```python
from build123d import *

# Parameters (mm, degrees)
SKETCH1_W               = 40
SKETCH1_H               = 20
BOSS_EXTRUDE1_DEPTH     = 36.6
SKETCH2_W               = 18
SKETCH2_H               = 2.6
BOSS_EXTRUDE2_DEPTH     = 7.25
SKETCH3_R               = 2.25
CUT_EXTRUDE1_DEPTH      = 42.17283692
MIRROR3_COPY_1_SKETCH_R = 2.25
MIRROR3_COPY_1_DEPTH    = 42.17283692
FILLET1_R               = 1
CHAMFER1_SIZE           = 1


with BuildPart() as part:
    # Sketch1 → Boss-Extrude1 (new body)
    with BuildSketch(Plane(origin=(0, 0, 0), x_dir=(1, 0, 0), z_dir=(0, 1, 0))):
        Rectangle(SKETCH1_W, SKETCH1_H)
    extrude(amount=BOSS_EXTRUDE1_DEPTH)

    # Sketch2 → Boss-Extrude2 (add)
    with BuildSketch(Plane(origin=(20, 0, 0), x_dir=(0, 0, -1), z_dir=(1, 0, 0))):
        with Locations((0, 27.9)):
            Rectangle(SKETCH2_W, SKETCH2_H)
    boss_extrude2 = extrude(amount=BOSS_EXTRUDE2_DEPTH)

    # Sketch3 → Cut-Extrude1 (cut, through all)
    with BuildSketch(Plane(origin=(0, 29.2, 0), x_dir=(1, 0, 0), z_dir=(0, 1, 0))):
        with Locations(Location((24.75, 5, 0), (0, 0, 270))):
            Circle(SKETCH3_R)
    cut_extrude1 = extrude(amount=-CUT_EXTRUDE1_DEPTH, mode=Mode.SUBTRACT)

    # Mirror2: Cut-Extrude1 across plane
    add(cut_extrude1.mirror(Plane.XY), mode=Mode.SUBTRACT)

    # Mirror3: Boss-Extrude2, Cut-Extrude1 across plane
    add(boss_extrude2.mirror(Plane(origin=(0, 0, 0), x_dir=(0, 0, 1), z_dir=(1, 0, 0))))
    add(cut_extrude1.mirror(Plane(origin=(0, 0, 0), x_dir=(0, 0, 1), z_dir=(1, 0, 0))), mode=Mode.SUBTRACT)

    # Mirror3 copy 1 sketch → Mirror3 copy 1 (cut, through all)
    with BuildSketch(Plane(origin=(0, 29.2, 0), x_dir=(-1, 0, 0), z_dir=(0, 1, 0))):
        with Locations(Location((24.75, 5, 0), (0, 0, 270))):
            Circle(MIRROR3_COPY_1_SKETCH_R)
    extrude(amount=-MIRROR3_COPY_1_DEPTH, mode=Mode.SUBTRACT)

    # Fillet1
    fillet1_edges = [part.edges().sort_by_distance(p)[0] for p in [
        (20, 18.3, 10),
        (-20, 18.3, 10),
        (-20, 18.3, -10),
        (20, 18.3, -10),
    ]]
    fillet(fillet1_edges, radius=FILLET1_R - 0.0001)  # a hair under: the kernel refuses the full size

    # Chamfer1
    chamfer1_edges = [part.edges().sort_by_distance(p)[0] for p in [
        (20, 0, 0),
        (0, 0, 10),
        (-20, 0, 0),
        (0, 0, -10),
        (-19.707136071, 0, 9.707136071),
        (-19.707136071, 0, -9.707136071),
        (19.707136071, 0, -9.707136071),
        (19.707136071, 0, 9.707136071),
    ]]
    chamfer(chamfer1_edges, length=CHAMFER1_SIZE - 0.0001)  # a hair under: the kernel refuses the full size


solid = part.part
```
Can you work these out from the model? Positions are in its coordinate system, mm. A direction names the side the tool comes from. Coordinates: 2 decimals unless noted, no trailing zeros. Loops run counter-clockwise (first coordinate to the right, second up) from the corner with the lowest first, then second, coordinate; pieces in that order, holes last.
Item 1: Please list where these lines run through material, in increasing order: L1, parallel to X at y = 27.85, z = 5; L2, parallel to Z at x = -24.75, y = 27.8; L3, parallel to Z at x = -24, y = 27.
Answers below:
L1: x = -27.25 to -27, -22.5 to 22.5, 27 to 27.25
L2: z = -9 to -7.25, -2.75 to 2.75, 7.25 to 9
L3: z = -9 to -7.12, -2.88 to 2.88, 7.12 to 9
Item 2: Suppose I cut it at C-C (y = 33.5). Please give me the cut outline in (x, z), then the cut area to 3 significant figures.
Answers below:
outline: (-20, -9) arc R1 ccw to (-19, -10) - (19, -10) arc R1 ccw to (20, -9) - (20, 9) arc R1 ccw to (19, 10) - (-19, 10) arc R1 ccw to (-20, 9) - close
area: 799 mm2
Item 3: I'm going to push flat-ended pins straight in: pin 1 (12 mm diameter, centred on y = 10, z = 6, fed in from +X); pin 2 (1 mm diameter, centred on y = 7.5, z = 1, fed in from -X); pin 3 (3.5 mm diameter, centred on x = -23, z = 3.5, fed in from +Y). Where does each tip first touch, or does it pass through?
Answers below:
pin 1: stops at x = 20
pin 2: stops at x = -20
pin 3: stops at y = 29.2
Item 4: Suppose I cut it at D-D (z = 0). Please give me the cut outline in (x, y).
Answers below:
outline: (-27.25, 26.6) - (-20, 26.6) - (-20, 1) - (-19, 0) - (19, 0) - (20, 1) - (20, 26.6) - (27.25, 26.6) - (27.25, 29.2) - (20, 29.2) - (20, 36.6) - (-20, 36.6) - (-20, 29.2) - (-27.25, 29.2) - close
Item 5: Suppose I cut it at A-A (z = -5). Please give me the cut outline in (x, y).
Answers below:
outline: (-27.25, 26.6) - (-27, 26.6) - (-27, 29.2) - (-27.25, 29.2) - close; (-22.5, 26.6) - (-20, 26.6) - (-20, 1) - (-19, 0) - (19, 0) - (20, 1) - (20, 26.6) - (22.5, 26.6) - (22.5, 29.2) - (20, 29.2) - (20, 36.6) - (-20, 36.6) - (-20, 29.2) - (-22.5, 29.2) - close; (27, 26.6) - (27.25, 26.6) - (27.25, 29.2) - (27, 29.2) - close
Item 6: Which directions (+Z, -Z, +X, -X, +Y, -Y) give clear straight access to the entire face, cutting with the end or side of a thin tool? Please do faces 4 (the face through (24, 28, -9)), 5 (the face through (24, 28, 9)), 6 (the face through (-24, 28, 9)), 7 (the face through (24, 29.2, 0)), 8 (the face through (-24, 29.2, 0)).
Answers below:
face 4: -Z, +X, +Y, -Y
face 5: +Z, +X, +Y, -Y
face 6: +Z, -X, +Y, -Y
face 7: +Z, -Z, +X, +Y
face 8: +Z, -Z, -X, +Y
Item 7: Suppose I cut it at B-B (x = 24.75). Please give me the cut outline in (y, z), then the cut area to 3 significant figures.
Answers below:
outline: (26.6, -9) - (29.2, -9) - (29.2, -7.25) - (26.6, -7.25) - close; (26.6, -2.75) - (29.2, -2.75) - (29.2, 2.75) - (26.6, 2.75) - close; (26.6, 7.25) - (29.2, 7.25) - (29.2, 9) - (26.6, 9) - close
area: 23.4 mm2
Item 8: If we mould it in two halves opening along X, with no side actions, what happens to faces 1 (the face through (0, 19, 10)), 2 (the face through (-20, 19, 0)), 3 (the face through (-22.554, 27.918, 5.488))? For each: released by +X, released by -X, zero draft, split by the parting line, or undercut.
Answers below:
face 1: zero draft
face 2: released by -X
face 3: undercut
